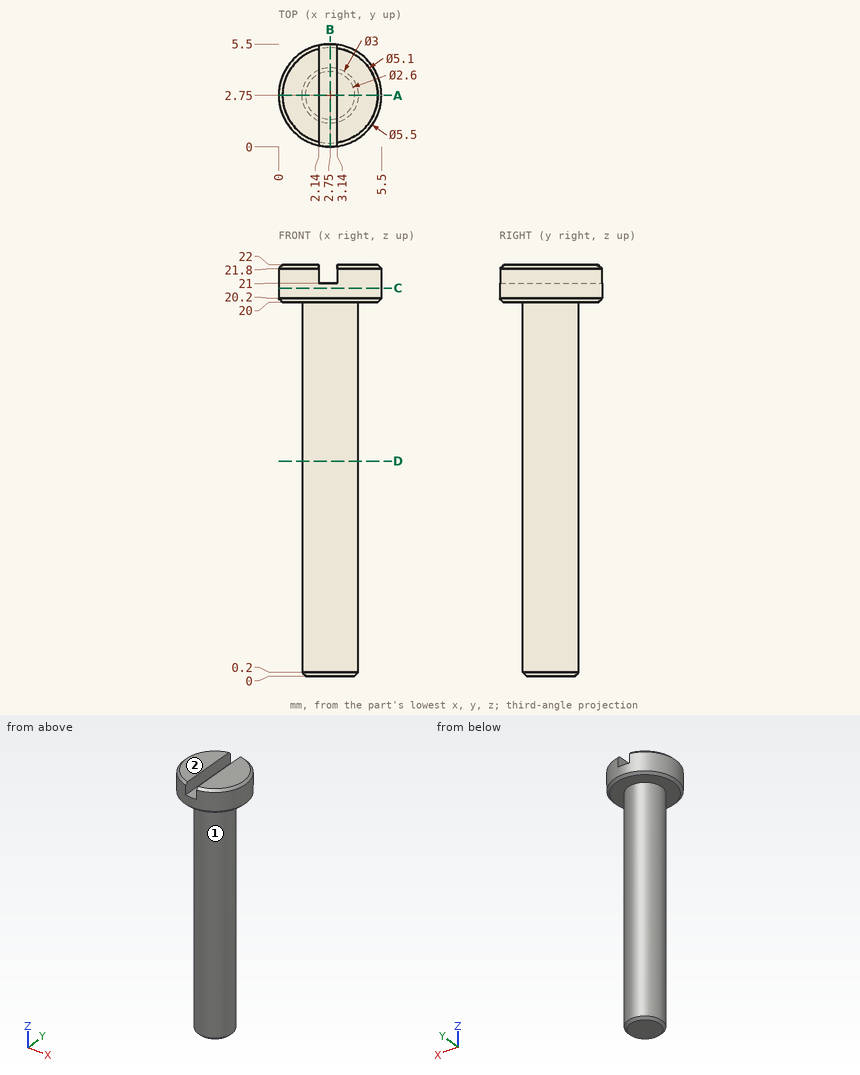
Design review of the part shown in the three views and the two pictorial views. Dimensions are in mm from the part's minimum x, y and z. A direction names the side the tool comes from. Round coordinates to 2 decimals unless told otherwise and drop trailing zeros. Write each loop counter-clockwise with the first axis right and the second up, starting at its lowest first coordinate (ties: lowest second). Pieces come first, ordered by that corner, then holes. Notation, with made-up numbers: (-15, 89.25) - (18, 89.25) arc R24 ccw to (18, 106.25) - close; hole circle Ø7 at (-15, 8). An arc over 180 degrees is marked (long way). Write item = value, one per line. Start each with the question number.
1. Consider section D-D on z = 11.5. State the section outline as (x, y) points.
2. Consider section C-C on z = 20.75. State the section outline as (x, y) points.
3. Wall thickness on L1, parallel to Z at x = 2.85, y = 2.35; L2, parallel to Z at x = 4.55, y = 2.35; L3, parallel to Y at x = 2.8, z = 11: over which ranges is each line inside the solid? List them lowest first.
4. For pin 1 Ø0.5 at (y, z) = (2, 21.5) entering from -X; pin 2 Ø2 at (y, z) = (3, 17.5) entering from -X, all flat-tipped, find the tip position at first contact; note any pin that passes through.
5. For the marked faces 1 and 2, list the 3-axis set-ups (+Z, -Z, +X, -X, +Y, -Y) from which the entire face can be reached by the end or side of a thin tool; tool diameter is ignored.
6. Consider section B-B on x = 2.75. State the section outline as (y, z) points.
7. Consider section A-A on y = 2.75. State the section outline as (x, z) points.
Evaluation:
q1.outline = circle Ø3 at (2.75, 2.75)
q2.outline = circle Ø5.5 at (2.75, 2.75)
q3.L1 = 0 to 21
q3.L2 = 20 to 22
q3.L3 = 1.25 to 4.25
q4.pin_1 = 0.05
q4.pin_2 = 1.25
q5.face_1 = -Z
q5.face_2 = +Z, +X, -X, +Y, -Y
q6.outline = (0, 20.2) - (0.2, 20) - (1.25, 20) - (1.25, 0.2) - (1.45, 0) - (4.05, 0) - (4.25, 0.2) - (4.25, 20) - (5.3, 20) - (5.5, 20.2) - (5.5, 21) - (0, 21) - close
q7.outline = (0, 20.2) - (0.2, 20) - (1.25, 20) - (1.25, 0.2) - (1.45, 0) - (4.05, 0) - (4.25, 0.2) - (4.25, 20) - (5.3, 20) - (5.5, 20.2) - (5.5, 21.8) - (5.3, 22) - (3.14, 22) - (3.14, 21) - (2.14, 21) - (2.14, 22) - (0.2, 22) - (0, 21.8) - close
